Job drawing, mm, ordinate dimensions from the low corner. One solid piece. A direction names the side the tool comes from. Give positions to 0.01 mm unless a question says otherwise; leave off trailing zeros. Loops run counter-clockwise (first coordinate to the right, second up) from the corner with the lowest first, then second, coordinate; pieces in that order, holes last.
Item 1: Saw through at B-B on x = 5. Give the cut face in (y, z).
Item 2: Probe probe 1 along X at (y, z) = (114.5, 5.5); probe 2 along Z at (x, y) = (34, 41.5) (1 decimal). List the from-to ranges inside material, lowest first.
Item 3: Saw through at C-C on z = 5.5. Give the cut face in (x, y).
Item 4: Saw through at A-A on y = 38. Give the cut face in (x, z).
Item 5: Drop flat-ended pins along their axis: P1, Ø10, axis at x = 36, y = 58.5, coming from the +Z side; P2, Ø4, axis at x = 42.5, y = 41.5, coming from the +Z side; P3, Ø4, axis at y = 62.5, z = 4, coming from the +X side. Give the stop position or say it passes through.
Item 6: Which spindle directions (+Z, -Z, +X, -X, +Y, -Y) get a long thin tool onto all of the face, cutting with end or side? Do the marked faces 1, 2 and 3. Say none if no direction does.
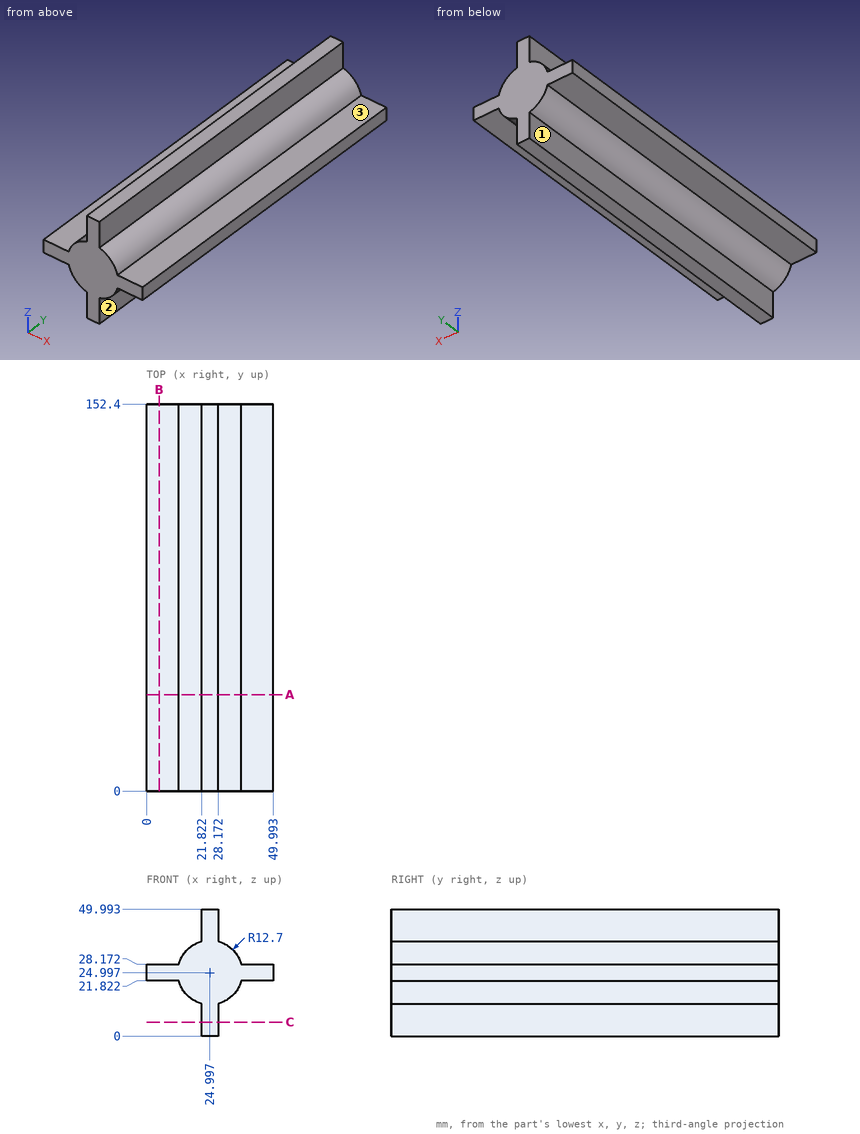
Results below:
1. outline: (0, 21.82) - (152.4, 21.82) - (152.4, 28.17) - (0, 28.17) - close
2. probe 1: x = 21.82 to 28.17
2. probe 2: z = 16 to 34
3. outline: (21.82, 0) - (28.17, 0) - (28.17, 152.4) - (21.82, 152.4) - close
4. outline: (0, 21.82) - (12.7, 21.82) arc R12.7 ccw to (21.82, 12.7) - (21.82, 0) - (28.17, 0) - (28.17, 12.7) arc R12.7 ccw to (37.29, 21.82) - (49.99, 21.82) - (49.99, 28.17) - (37.29, 28.17) arc R12.7 ccw to (28.17, 37.29) - (28.17, 49.99) - (21.82, 49.99) - (21.82, 37.29) arc R12.7 ccw to (12.7, 28.17) - (0, 28.17) - close
5. P1: stops at z = 36.19
5. P2: stops at z = 28.17
5. P3: stops at x = 28.17
6. face 1: -Z, -X, +Y, -Y
6. face 2: -Z, +X, +Y, -Y
6. face 3: +Z, +X, +Y, -Y
